CAD build for the part. Positions are in the model's coordinates, mm. Face numbers are marked on the shaded views. Round coordinates to 2 decimals unless told otherwise and drop trailing zeros. Order: outer loops, then holes, each group sorted by start corner. A loop starts at its lowest first (then second) coordinate and runs counter-clockwise, first axis right, second up. Notation, with made-up numbers: (2, -27.5) -> (12, -27.5) arc R27 ccw to (12, 4.5) -> close; hole circle Ø9 at (-29.5, 64.5). An arc over 180 degrees is marked (long way). Return JSON: item names as keys, results as strings. Group by question number.
Q1. Mould opens along Y. For the marked faces 1, 2 and 3 say: +Y half, -Y half, draft (parallel to the pull), parting line (faces both ways), or undercut.
Q2. Cut at B-B (y = -18). Write the cut outline in (x, z), then the cut area to 3 significant figures.
Q3. Cut at A-A (z = 12.5). Write the cut outline in (x, y), then the cut area to 3 significant figures.
Q4. Probe line 1 along Z through (x, y) = (-49, -41); line 2 along Y through (x, z) = (2, 8). List the from-to ranges inside material, lowest first.
Q5. Cut at C-C (x = -6). Write the cut outline in (y, z), then the cut area to 3 significant figures.
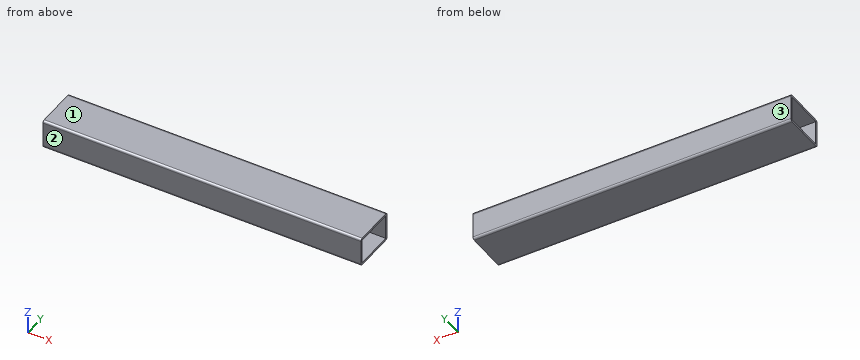
from build123d import *

# Parameters (mm, degrees)
F0_W     = 54
F0_H     = 34
F1_DEPTH = 219


with BuildPart() as f1:
    # F0 (on Right) → F1 (new body, symmetric)
    with BuildSketch(Plane.YZ):
        with BuildLine():
            ThreePointArc((3, 34), (2.12132, 36.12132), (0, 37))
            Line((0, 37), (-54, 37))
            ThreePointArc((-54, 37), (-56.12132, 36.12132), (-57, 34))
            Line((-57, 34), (-57, 0))
            ThreePointArc((-57, 0), (-56.12132, -2.12132), (-54, -3))
            Line((-54, -3), (0, -3))
            ThreePointArc((0, -3), (2.12132, -2.12132), (3, 0))
            Line((3, 0), (3, 34))
        make_face()
        with Locations((-27, 17)):
            Rectangle(F0_W, F0_H, mode=Mode.SUBTRACT)
    extrude(amount=F1_DEPTH, both=True)


solid = f1.part
Solution:
{
 "1": {"face 1": "draft", "face 2": "-Y half", "face 3": "+Y half"},
 "2": {"outline": "(-219, -3) -> (219, -3) -> (219, 0) -> (-219, 0) -> close; (-219, 34) -> (219, 34) -> (219, 37) -> (-219, 37) -> close", "area": "2,630 mm²"},
 "3": {"outline": "(-219, -57) -> (219, -57) -> (219, -54) -> (-219, -54) -> close; (-219, 0) -> (219, 0) -> (219, 3) -> (-219, 3) -> close", "area": "2,630 mm²"},
 "4": {"line 1": "z = -3 to 0, 34 to 37", "line 2": "y = -57 to -54, 0 to 3"},
 "5": {"outline": "(-57, 0) arc R3 ccw to (-54, -3) -> (0, -3) arc R3 ccw to (3, 0) -> (3, 34) arc R3 ccw to (0, 37) -> (-54, 37) arc R3 ccw to (-57, 34) -> close; hole (-54, 0) -> (0, 0) -> (0, 34) -> (-54, 34) -> close", "area": "556 mm²"}
}
